Read the model definition and answer for the solid it produces. Units are mm, in the model's axes. A direction names the side the tool comes from. Round coordinates to 2 decimals unless told otherwise and drop trailing zeros. Loops run counter-clockwise (first coordinate to the right, second up) from the corner with the lowest first, then second, coordinate; pieces in that order, holes last. Notation, with made-up numbers: M 57.25,-9 L 114.25,-9 A24 cw 114.25,4 Z; hole C 70.25,55.25 d7. An arc over 180 degrees is marked long. Write each question's results on one line, items separated by ' | '.
```python
from build123d import *

# Parameters (mm, degrees)
SKETCH_W     = 19.2
SKETCH_H     = 19.2
PAD_DEPTH    = 2
PAD001_DEPTH = 8
FILLET_R     = 1
SKETCH012_R  = 5
PAD002_DEPTH = 10
POCKET_DEPTH = 10


with BuildPart() as part:
    # Sketch → Pad (new body)
    with BuildSketch(Plane.XY):
        Rectangle(SKETCH_W, SKETCH_H)
    extrude(amount=PAD_DEPTH)

    # Sketch011 → Pad001 (new body)
    with BuildSketch(Plane.XY.offset(2)):
        Polygon((-9.6, 7.125126), (-7.125126, 9.6), (-9.6, 9.6), align=None)
        Polygon((7.125126, 9.6), (9.6, 9.6), (9.6, 7.125126), align=None)
        Polygon((7.125126, -9.6), (9.6, -9.6), (9.6, -7.125126), align=None)
        Polygon((-7.125126, -9.6), (-9.6, -9.6), (-9.6, -7.125126), align=None)
    extrude(amount=PAD001_DEPTH)

    # Fillet
    fillet_edges = [part.edges().sort_by_distance(p)[0] for p in [
        (-8.362563, 8.362563, 2),
        (8.362563, 8.362563, 2),
        (8.362563, -8.362563, 2),
        (-8.362563, -8.362563, 2),
    ]]
    fillet(fillet_edges, radius=FILLET_R)

    # Sketch012 → Pad002 (new body)
    with BuildSketch(Plane(origin=(0, 0, 0), x_dir=(1, 0, 0), z_dir=(0, 0, -1))):
        Circle(SKETCH012_R)
    extrude(amount=PAD002_DEPTH)

    # Sketch008 → Pocket (cut)
    with BuildSketch(Plane(origin=(0, 0, -10), x_dir=(1, 0, 0), z_dir=(0, 0, -1))):
        with BuildLine():
            Line((-1.684191, 2.02), (1.684191, 2.02))
            ThreePointArc((-1.684191, 2.02), (0, -2.63), (1.684191, 2.02))
        make_face()
    extrude(amount=-POCKET_DEPTH, mode=Mode.SUBTRACT)


solid = part.part
```
1. Find section B-B, the plane x = 0. Give the vertices of the cut face in (y, z).
Completed:
outline: M -9.6,0 L -5,0 L -5,-10 L -2.02,-10 L -2.02,0 L 2.63,0 L 2.63,-10 L 5,-10 L 5,0 L 9.6,0 L 9.6,2 L -9.6,2 Z
2. Find the intervals of material crossed by L1, parallel to X at y = 0, z = -5.5; L2, parallel to Y at x = 0, z = -2.5; L3, parallel to Z at x = 0.75, y = -5, in increasing order.
Completed:
L1: x = -5 to -2.63, 2.63 to 5 | L2: y = -5 to -2.02, 2.63 to 5 | L3: z = 0 to 2
3. Determine the mould class of faces 1 (the face through (-9, 9, 10)), 2 (the face through (-8.38, 8.345, 6.451)), 3 (the face through (0.1, 9.6, 1.6)), 4 (the face through (0, -2.02, -5)) for opening direction Y: released by +Y, released by -Y, zero draft, split by the parting line, or undercut.
Completed:
face 1: zero draft | face 2: undercut | face 3: released by +Y | face 4: undercut
4. Find section C-C, the plane z = -2.5. Give the vertices of the cut face in (x, y).
Completed:
outline: C 0,0 d10; hole M -1.68,-2.02 L 1.68,-2.02 A2.63 ccw long Z
5. Given P1, Ø4, axis at y = 5, z = 7.5, coming from the -X side; P2, Ø3.5, axis at x = -0.5, z = -3, coming from the +Y side; P3, Ø8, axis at x = 3.5, y = 3, coming from the +Z side; P4, Ø1.4, axis at x = -0.5, y = 1.5, coming from the -Z side, each flat-ended and moving along its own axis, determine where each tip first touches the part or whether it passes through.
Completed:
P1: passes through | P2: stops at y = 5 | P3: stops at z = 2 | P4: stops at z = 0
6. Which of the six approach directions +Z, -Z, +X, -X, +Y, -Y give full straight-line access (tool end or side, diameter ignored) to faces 5 (the face through (9, 9, 10)), 6 (the face through (4, 4, 0)), 7 (the face through (8.027, 8.082, 2.175))?
Completed:
face 5: +Z, +X, -X, +Y, -Y | face 6: -Z | face 7: +Z
7. Find section A-A, the plane y = 0. Give the vertices of the cut face in (x, z).
Completed:
outline: M -9.6,0 L -5,0 L -5,-10 L -2.63,-10 L -2.63,0 L 2.63,0 L 2.63,-10 L 5,-10 L 5,0 L 9.6,0 L 9.6,2 L -9.6,2 Z
8. Find section D-D, the plane x = -3.5. Give the vertices of the cut face in (y, z).
Completed:
outline: M -9.6,0 L -3.57,0 L -3.57,-10 L 3.57,-10 L 3.57,0 L 9.6,0 L 9.6,2 L -9.6,2 Z
